Design review of the part built by this model. Coordinates are the model's own, in mm. Coordinates: 2 decimals unless noted, no trailing zeros. Write each loop counter-clockwise with the first axis right and the second up, starting at its lowest first coordinate (ties: lowest second). Pieces come first, ordered by that corner, then holes.
Q1. Mouldability with a two-part tool opening along X and no side actions: class faces 1 (the cylindrical face through (-12.71, 39.04, -8.52)), 2 (the cylindrical face through (15.096, 39.042, -7.652)), 3 (the cylindrical face through (-39.04, 12.8, -8.85)) as pulls with the +X half, pulls with the -X half, needs draft (parallel to the pull), parting line crosses it, or undercut.
Q2. Take a section at B-B (y = -27). Give the boundary of the cut face in (x, z), and give its area (3 significant figures).
Q3. Insertion check: pin 1 (4 mm diameter, centred on x = 33.95, y = -33.95, fed in from +Z); pin 2 (2 mm diameter, centred on x = -14, z = -8.35, fed in from -Y); pin 3 (3.5 mm diameter, centred on x = -33.95, y = -33.95, fed in from -Z). Each pin has a flat end and moves straight along its axis. Give the tip position at first contact, or say it passes through.
Q4. Take a section at A-A (x = 22.5). Give the boundary of the cut face in (y, z), and give its area (3 significant figures).
Q5. For probe 1 along Y at (x, z) = (-26, -5.5); probe 2 along Z at (x, y) = (-0.5, -33.5), list the stretches that pass through material, from the lowest coordinate up.
```python
from build123d import *

# Parameters (mm, degrees)
PAD015_DEPTH         = 84
SKETCH025_R          = 3
POCKET009_DEPTH      = 3.1
SKETCH026_R          = 1.55
POCKET010_DEPTH      = 3.9054430506
SKETCH029_R          = 1.3
POCKET013_DEPTH      = 5.0055349839
SKETCH036_R          = 1.3
POCKET018_DEPTH      = 7.0054430506
SKETCH040_R          = 1.3
POCKET021_DEPTH      = 7.0054430506
POCKET021_FACE10_W   = 84
POCKET021_FACE10_H   = 84
POCKET021_FACE10_R   = 1.3
POCKET021_FACE10_R_2 = 3
PAD021_DEPTH         = 1.25
SKETCH041_R          = 1.3
POCKET022_DEPTH      = 6
SKETCH042_R          = 1.3
POCKET023_DEPTH      = 6
SKETCH043_R          = 1.3
POCKET024_DEPTH      = 6
SKETCH044_R          = 1.3
POCKET025_DEPTH      = 6


with BuildPart() as part:
    # Sketch024 (on DatumPlane) → Pad015 (new body)
    with BuildSketch(Plane(origin=(42.0007630338, 0.0001547258, 16.9985727734), x_dir=(0, -1, 9.1023e-06), z_dir=(0.999999999, -4e-10, -4.48856e-05))):
        Polygon((-42, 22.85), (-31.9, 22.85), (-31.9, 20.85), (-28.1, 20.85), (-28.1, 22.85), (28.1, 22.85), (28.1, 20.85), (31.9, 20.85), (31.9, 22.85), (42, 22.85), (42, 27.85), (-42, 27.85), align=None)
    extrude(amount=-PAD015_DEPTH)

    # Sketch025 (on Face11 of Pad015) → Pocket009 (cut)
    with BuildSketch(Plane(origin=(41.9995129693, -9.87728e-05, -10.8514271974), x_dir=(0, 1, -9.1023e-06), z_dir=(-4.48856e-05, -9.1023e-06, -0.999999999))):
        with Locations((-12.5, -10)):
            Circle(SKETCH025_R)
        with Locations((12.5, -10)):
            Circle(SKETCH025_R)
    extrude(amount=-POCKET009_DEPTH, mode=Mode.SUBTRACT)

    # Sketch026 (on Face17 of Pocket009) → Pocket010 (cut, through all)
    with BuildSketch(Plane(origin=(41.9996521147, -7.05557e-05, -7.7514272007), x_dir=(0, 1, -9.1023e-06), z_dir=(-4.48856e-05, -9.1023e-06, -0.999999999))):
        with Locations((-12.5, -10)):
            Circle(SKETCH026_R)
        with Locations((12.5, -10)):
            Circle(SKETCH026_R)
    extrude(amount=-POCKET010_DEPTH, mode=Mode.SUBTRACT)

    # Sketch029 (on Face13 of Pocket010) → Pocket013 (cut, through all)
    with BuildSketch(Plane(origin=(41.9997373974, -5.32613e-05, -5.8514272027), x_dir=(0, -1, 9.1023e-06), z_dir=(4.48856e-05, 9.1023e-06, 0.999999999))):
        with Locations((37, -5)):
            Circle(SKETCH029_R)
        with Locations((-37, -5)):
            Circle(SKETCH029_R)
    extrude(amount=-POCKET013_DEPTH, mode=Mode.SUBTRACT)

    # Sketch036 (on Face7 of Pocket013) → Pocket018 (cut, through all)
    with BuildSketch(Plane(origin=(41.9995129693, -9.87728e-05, -10.8514271974), x_dir=(0, 1, -9.1023e-06), z_dir=(-4.48856e-05, -9.1023e-06, -0.999999999))):
        with Locations((-37, -79)):
            Circle(SKETCH036_R)
        with Locations((37, -79)):
            Circle(SKETCH036_R)
    extrude(amount=-POCKET018_DEPTH, mode=Mode.SUBTRACT)

    # Sketch040 (on Face8 of Pocket018) → Pocket021 (cut, through all)
    with BuildSketch(Plane(origin=(41.9995129693, -9.87728e-05, -10.8514271974), x_dir=(0, 1, -9.1023e-06), z_dir=(-4.48856e-05, -9.1023e-06, -0.999999999))):
        with Locations((-33.95, -8.05)):
            Circle(SKETCH040_R)
        with Locations((-33.95, -75.95)):
            Circle(SKETCH040_R)
        with Locations((33.95, -75.95)):
            Circle(SKETCH040_R)
        with Locations((33.95, -8.05)):
            Circle(SKETCH040_R)
    extrude(amount=-POCKET021_DEPTH, mode=Mode.SUBTRACT)

    # Pocket021 Face10 → Pad021 (add)
    with BuildSketch(Plane(origin=(-0.2605938375, -9.87555e-05, -10.8495303264), x_dir=(0, -1, 9.1023e-06), z_dir=(-4.48856e-05, -9.1023e-06, -0.999999999))):
        with Locations((0, -0.2601068494)):
            Rectangle(POCKET021_FACE10_W, POCKET021_FACE10_H)
        with Locations((37, 36.7398931506)):
            Circle(POCKET021_FACE10_R, mode=Mode.SUBTRACT)
        with Locations((33.95, 33.6898931506)):
            Circle(POCKET021_FACE10_R, mode=Mode.SUBTRACT)
        with Locations((-37, 36.7398931506)):
            Circle(POCKET021_FACE10_R, mode=Mode.SUBTRACT)
        with Locations((-33.95, 33.6898931506)):
            Circle(POCKET021_FACE10_R, mode=Mode.SUBTRACT)
        with Locations((33.95, -34.2101068494)):
            Circle(POCKET021_FACE10_R, mode=Mode.SUBTRACT)
        with Locations((37, -37.2601068494)):
            Circle(POCKET021_FACE10_R, mode=Mode.SUBTRACT)
        with Locations((12.5, -32.2601068494)):
            Circle(POCKET021_FACE10_R_2, mode=Mode.SUBTRACT)
        with Locations((-12.5, -32.2601068494)):
            Circle(POCKET021_FACE10_R_2, mode=Mode.SUBTRACT)
        with Locations((-33.95, -34.2101068494)):
            Circle(POCKET021_FACE10_R, mode=Mode.SUBTRACT)
        with Locations((-37, -37.2601068494)):
            Circle(POCKET021_FACE10_R, mode=Mode.SUBTRACT)
    extrude(amount=PAD021_DEPTH)

    # Sketch041 (on Face16 of Pad021) → Pocket022 (cut)
    with BuildSketch(Plane(origin=(42.0007630338, 0.0001547258, 16.9985727734), x_dir=(0, -1, 9.1023e-06), z_dir=(0.999999999, -4e-10, -4.48856e-05))):
        with Locations((-14, 25.35)):
            Circle(SKETCH041_R)
        with Locations((14, 25.35)):
            Circle(SKETCH041_R)
    extrude(amount=-POCKET022_DEPTH, mode=Mode.SUBTRACT)

    # Sketch042 (on Face12 of Pocket022) → Pocket023 (cut)
    with BuildSketch(Plane(origin=(42.0007630338, -41.9998452724, 16.9989550693), x_dir=(-4.48856e-05, -9.1023e-06, -0.999999999), z_dir=(0, -1, 9.1023e-06))):
        with Locations((25.35, -28)):
            Circle(SKETCH042_R)
        with Locations((25.35, -56)):
            Circle(SKETCH042_R)
    extrude(amount=-POCKET023_DEPTH, mode=Mode.SUBTRACT)

    # Sketch043 (on Face4 of Pocket023) → Pocket024 (cut)
    with BuildSketch(Plane(origin=(-41.9992368816, 0.0001547602, 17.0023431654), x_dir=(0, -1, 9.1023e-06), z_dir=(-0.999999999, 4e-10, 4.48856e-05))):
        with Locations((-14, -25.35)):
            Circle(SKETCH043_R)
        with Locations((14, -25.35)):
            Circle(SKETCH043_R)
    extrude(amount=-POCKET024_DEPTH, mode=Mode.SUBTRACT)

    # Sketch044 (on Face2 of Pocket024) → Pocket025 (cut)
    with BuildSketch(Plane(origin=(42.0007630338, 42.0001547241, 16.9981904774), x_dir=(4.48856e-05, 9.1023e-06, 0.999999999), z_dir=(0, 1, -9.1023e-06))):
        with Locations((-25.35, -28)):
            Circle(SKETCH044_R)
        with Locations((-25.35, -56)):
            Circle(SKETCH044_R)
    extrude(amount=-POCKET025_DEPTH, mode=Mode.SUBTRACT)


solid = part.part
```
Response:
1. face 1: undercut
1. face 2: undercut
1. face 3: needs draft
2. outline: (-42, -12.1) - (42, -12.1) - (42, -5.85) - (-42, -5.85) - close
2. area: 525 mm2
3. pin 1: stops at z = -5.85
3. pin 2: stops at y = -36
3. pin 3: stops at z = -12.1
4. outline: (-42, -12.1) - (42, -12.1) - (42, -5.85) - (31.9, -5.85) - (31.9, -3.85) - (28.1, -3.85) - (28.1, -5.85) - (-28.1, -5.85) - (-28.1, -3.85) - (-31.9, -3.85) - (-31.9, -5.85) - (-42, -5.85) - close
4. area: 540 mm2
5. probe 1: y = -31.9 to -28.1, 28.1 to 31.9
5. probe 2: z = -12.1 to -5.85
